from build123d import *

# Parameters (mm, degrees)
F0_R     = 1.5875
F0_R_2   = 7.90575
F1_DEPTH = 9.525
F2_R     = 3.4925
F2_R_2   = 1.5875
F3_DEPTH = 6.35


with BuildPart() as f1:
    # F0 (on Top) → F1 (new body)
    with BuildSketch(Plane.XY):
        with BuildLine():
            Line((25.4, 22.606), (0, 22.606))
            ThreePointArc((0, 22.606), (-9.906, 12.7), (0, 2.794))
            Line((0, 2.794), (25.4, 2.794))
            ThreePointArc((25.4, 2.794), (35.306, 12.7), (25.4, 22.606))
        make_face()
        with Locations((-4.480041, 12.7)):
            Circle(F0_R, mode=Mode.SUBTRACT)
        with Locations((12.7, 12.7)):
            Circle(F0_R_2, mode=Mode.SUBTRACT)
        with Locations((28.654418, 12.7)):
            Circle(F0_R, mode=Mode.SUBTRACT)
    extrude(amount=F1_DEPTH)

    # F2 (on face) → F3 (cut)
    with BuildSketch(Plane.XY.offset(9.525)):
        with Locations((-4.480041, 12.7)):
            Circle(F2_R)
        with Locations((-4.480041, 12.7)):
            Circle(F2_R_2, mode=Mode.SUBTRACT)
        with Locations((28.654418, 12.7)):
            Circle(F2_R)
        with Locations((28.654418, 12.7)):
            Circle(F2_R_2, mode=Mode.SUBTRACT)
    extrude(amount=-F3_DEPTH, mode=Mode.SUBTRACT)


solid = f1.part
The listing builds one solid part. Answer for the finished solid, in the listing's coordinates (mm). A direction names the side the tool comes from. Coordinates: 2 decimals unless noted, no trailing zeros. Write each loop counter-clockwise with the first axis right and the second up, starting at its lowest first coordinate (ties: lowest second). Pieces come first, ordered by that corner, then holes. Notation, with made-up numbers: (80.25, -9.5) - (132.25, -9.5) arc R14 ccw to (132.25, 5.5) - close; hole circle Ø1 at (1.25, 59.25). An arc over 180 degrees is marked (long way). Put each result on its own line as item: value.
1. Flat-ended cylindrical pins translate along their axes: pin 1 Ø3 at (x, y) = (-4.48, 12.7) entering from -Z; pin 2 Ø5.5 at (x, y) = (-4.48, 12.7) entering from +Z (3 decimals). Find the tip coordinate at first contact, or state that the pin passes through.
Answer sheet:
pin 1: passes through
pin 2: stops at z = 3.175
2. Find the intervals of material crossed by line 1 along X through (y, z) = (15.75, 6.25); line 2 along Z through (x, y) = (31, 14.25) (3 decimals); line 3 along Y through (x, z) = (30.5, 5), in increasing order. Write a range as from..to.
Answer sheet:
line 1: x = -9.42..-6.18, -2.78..5.41, 19.99..26.95, 30.36..34.82
line 2: z = 0..3.175
line 3: y = 4.21..9.73, 15.67..21.19
3. Determine the mould class of faces 1 (the face through (35.304, 12.482, 4.696)), 2 (the face through (6.87, 18.04, 4.7)), 3 (the face through (13, 22.606, 5)) for opening direction X: pulls with the +X half, pulls with the -X half, needs draft (parallel to the pull), parting line crosses it, or undercut.
Answer sheet:
face 1: pulls with the +X half
face 2: undercut
face 3: needs draft
4. The part is cut by section C-C on z = 4. Give the vertices of the cut face in (x, y) (1 decimal).
Answer sheet:
outline: (0, 2.8) - (25.4, 2.8) arc R9.9 ccw to (25.4, 22.6) - (0, 22.6) arc R9.9 ccw to start; hole circle Ø7 at (-4.5, 12.7); hole circle Ø15.8 at (12.7, 12.7); hole circle Ø7 at (28.7, 12.7)
5. The part is cut by section B-B on y = 12.7. Give the vertices of the cut face in (x, z) (3 decimals), plus the area to 3 significant figures.
Answer sheet:
outline: (-9.906, 0) - (-6.068, 0) - (-6.068, 3.175) - (-7.973, 3.175) - (-7.973, 9.525) - (-9.906, 9.525) - close; (-2.893, 0) - (4.794, 0) - (4.794, 9.525) - (-0.988, 9.525) - (-0.988, 3.175) - (-2.893, 3.175) - close; (20.606, 0) - (27.067, 0) - (27.067, 3.175) - (25.162, 3.175) - (25.162, 9.525) - (20.606, 9.525) - close; (30.242, 0) - (35.306, 0) - (35.306, 9.525) - (32.147, 9.525) - (32.147, 3.175) - (30.242, 3.175) - close
area: 171 mm^2
6. The part is cut by section A-A on x = 12.7. Give the vertices of the cut face in (y, z) (3 decimals), plus the area to 3 significant figures.
Answer sheet:
outline: (2.794, 0) - (4.794, 0) - (4.794, 9.525) - (2.794, 9.525) - close; (20.606, 0) - (22.606, 0) - (22.606, 9.525) - (20.606, 9.525) - close
area: 38.1 mm^2
7. The part is cut by section D-D on y = 18. Give the vertices of the cut face in (x, z) (3 decimals), plus the area to 3 significant figures.
Answer sheet:
outline: (-8.369, 0) - (6.834, 0) - (6.834, 9.525) - (-8.369, 9.525) - close; (18.566, 0) - (33.769, 0) - (33.769, 9.525) - (18.566, 9.525) - close
area: 290 mm^2
8. A tool of negligible diameter and unlimited length cuts with its end or side. For faces 4 (the face through (28, 11, 3.175)), 5 (the face through (30.169, 13.177, 1.565)), from which of +Z, -Z, +X, -X, +Y, -Y can it reach the whole face along a straight path? Write none if from no direction.
Answer sheet:
face 4: +Z
face 5: +Z, -Z
